Model file for the job. Use its own axes, mm. A direction names the side the tool comes from. Give positions to 0.01 mm unless a question says otherwise; leave off trailing zeros. Write each loop counter-clockwise with the first axis right and the second up, starting at its lowest first coordinate (ties: lowest second). Pieces come first, ordered by that corner, then holes.
Autodesk Inventor part; units mm, degrees
ref_plane "YZ Plane" through (0, 0, 0) normal (1, 0, 0) x (0, 1, 0)
ref_plane "XZ Plane" through (0, 0, 0) normal (0, 1, 0) x (-1, 0, 0)
ref_plane "XY Plane" through (0, 0, 0) normal (0, 0, 1) x (1, 0, 0)
sketch "Sketch1" plane through (0, 0, 0) normal (1, 0, 0) x (0, 1, 0)
  line L0 (-243.5, 137) -> (243.5, 137)
  line L1 (243.5, 137) -> (243.5, -137)
  line L2 (243.5, -137) -> (-243.5, -137)
  line L3 (-243.5, -137) -> (-243.5, 137)
  line L4 (-243.5, 137) -> (243.5, -137) construction
  line L5 (243.5, 137) -> (-243.5, -137) construction
  line L6 (263.5, -157) -> (263.5, 157)
  line L7 (263.5, 157) -> (-263.5, 157)
  line L8 (-263.5, 157) -> (-263.5, -157)
  line L9 (-263.5, -157) -> (263.5, -157)
  point P0 (0, 0)
  dimension "d0" = 487
  dimension "d1" = 274
  dimension "d2" = 20
extrude "Extrusion1" add sketch "Sketch1" along normal blind 20 contours L0 L1 L2 L3 | L9 L8 L7 L6
extrude "Extrusion2" cut sketch "Sketch1" along normal blind 2 contours L0 L1 L2 L3
sketch "Sketch2" plane through (20, 0, 0) normal (1, 0, 0) x (0, 0, -1)
  line L0 (-157, 263.5) -> (-157, -263.5)
  line L1 (-157, -263.5) -> (157, -263.5)
  line L2 (157, -263.5) -> (157, 263.5)
  line L3 (157, 263.5) -> (-157, 263.5)
  line L4 (-107, 213.5) -> (-107, -213.5)
  line L5 (-107, -213.5) -> (107, -213.5)
  line L6 (107, -213.5) -> (107, 213.5)
  line L7 (107, 213.5) -> (-107, 213.5)
  point P0 (0, 0)
  dimension "d7" = 50
extrude "Extrusion3" add sketch "Sketch2" along normal blind 30 contours L7 L6 L5 L4
chamfer "Chamfer1" distance 25 angle 45 4 edges at (20, 0, -107) (50, 213.5, 0) (20, 0, 107) (20, -213.5, 0)
properties part number "DIMENSIONES_PANTALLA" material "Steel, Mild, Welded"
1. Pin check, flat tips, straight feed: P1, Ø5, axis at y = -55, z = -99, coming from the -X side; P2, Ø2.5, axis at x = 46.5, y = 12, coming from the -Z side; P3, Ø1.5, axis at x = 48, y = -85, coming from the +Z side. Stop position of each tip, or through.
Calculated:
P1: stops at x = 2
P2: stops at z = -107
P3: stops at z = 107
2. Pull direction Y, two halves, no side cores. Call faces 1 (the flat face through (32.7, -225.8, 1.8)), 2 (the flat face through (37.7, 200.8, 1.8)), 3 (the flat face through (2, -3, 2)), 4 (the flat face through (10, 4, 157)): +Y half, -Y half, draft (parallel to the pull), parting line (faces both ways), or undercut.
Calculated:
face 1: -Y half
face 2: +Y half
face 3: undercut
face 4: draft
3. Slice it at C-C, the plane x = 32.5. Write the cut outline in (y, z).
Calculated:
outline: (-226, -119.5) - (206, -119.5) - (206, 119.5) - (-226, 119.5) - close
4. Slice it at B-B, the plane y = 165. Write the cut outline in (x, z).
Calculated:
outline: (0, -157) - (20, -157) - (20, -132) - (45, -107) - (50, -107) - (50, 107) - (45, 107) - (20, 132) - (20, 157) - (0, 157) - (0, 137) - (2, 137) - (2, -137) - (0, -137) - close
5. Which spindle directions (+Z, -Z, +X, -X, +Y, -Y) get a long thin tool onto all of the face, cutting with end or side? Do faces 5 (the flat face through (0, -21, -139)), 6 (the flat face through (20, 57, -139)). Say none if no direction does.
Calculated:
face 5: +Z, -Z, -X, +Y, -Y
face 6: +X
6. Probe probe 1 along X at (y, z) = (-170.5, 91); probe 2 along X at (y, z) = (162, 139); probe 3 along Y at (x, z) = (43.5, 44.5). List the from-to ranges inside material, lowest first.
Calculated:
probe 1: x = 2 to 50
probe 2: x = 0 to 20
probe 3: y = -215 to 195
7. Slice it at A-A, the plane z = -56. Write the cut outline in (x, y), and give its area (3 significant figures).
Calculated:
outline: (0, -263.5) - (20, -263.5) - (20, -238.5) - (45, -213.5) - (50, -213.5) - (50, 188.5) - (25, 213.5) - (20, 213.5) - (20, 263.5) - (0, 263.5) - (0, 243.5) - (2, 243.5) - (2, -243.5) - (0, -243.5) - close
area: 22,400 mm2
